Geometry: final body of the model. Coordinates: model frame, mm. Face numbers are marked on the shaded views. Round coordinates to 2 decimals unless told otherwise and drop trailing zeros. Order: outer loops, then holes, each group sorted by start corner. A loop starts at its lowest first (then second) coordinate and runs counter-clockwise, first axis right, second up. Notation, with made-up numbers: (-4, -3.75) -> (4, -3.75) arc R28 cw to (4, 17.25) -> close; hole circle Ø3 at (56.25, -30.75). An arc over 180 degrees is marked (long way). Put each result on its own line as item: value.
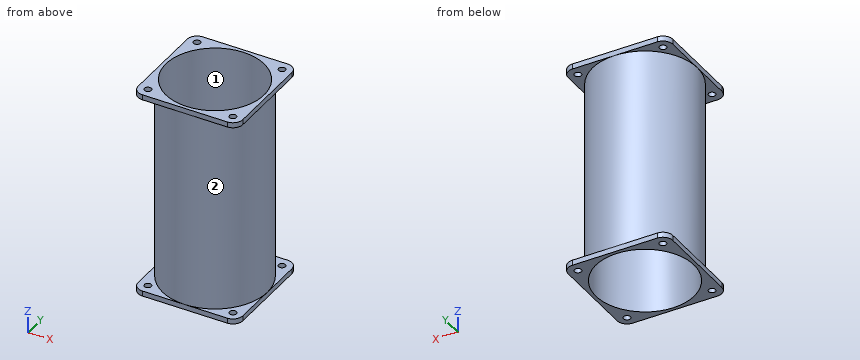
Autodesk Inventor part; units mm, degrees
ref_plane "YZ Plane" through (0, 0, 0) normal (1, 0, 0) x (0, 1, 0)
ref_plane "XZ Plane" through (0, 0, 0) normal (0, 1, 0) x (-1, 0, 0)
ref_plane "XY Plane" through (0, 0, 0) normal (0, 0, 1) x (1, 0, 0)
sketch "Skizze1" plane through (0, 0, 0) normal (0, 1, 0) x (-1, 0, 0)
  line L0 (0, 0) -> (80, 0)
  line L1 (80, 0) -> (80, -152)
  line L2 (80, -152) -> (0, -152)
  line L3 (0, -152) -> (0, 0)
  line L4 (80, -152) -> (-80, -152)
  line L5 (-80, -152) -> (-80, -160)
  line L6 (-80, -160) -> (80, -160)
  line L7 (80, -160) -> (80, -152)
  dimension "d0" = 160
  dimension "d1" = 160
  dimension "d2" = 8
revolve "Umdrehung1" add sketch "Skizze1" angle 360 about axis through (0, 0, -152) along (0, 0, 1) contours L0 L1 L2 L3
extrude "Extrusion1" add sketch "Skizze1" along normal mid plane 160 contours L2 L7 L6 L5 L4
fillet "Rundung1" radius 15 4 edges at (80, 80, -156) (-80, 80, -156) (80, -80, -156) (-80, -80, -156)
sketch "Skizze2" plane through (65, 80, -160) normal (0, 0, -1) x (-1, 0, 0)
  circle A0 centre (65, -80) radius 80
hole "Bohrung1" at (0, 0, -160) direction (0, 0, 1) diameter 150 end through all
sketch "Skizze3" plane through (65, 80, -160) normal (0, 0, -1) x (-1, 0, 0)
  line L0 (130, -145) -> (0, -145)
  line L1 (0, -145) -> (0, -15)
  line L2 (0, -15) -> (130, -15)
  line L3 (130, -15) -> (130, -145)
  line L4 (130, -145) -> (0, -15) construction
  line L5 (0, -145) -> (130, -15) construction
  point P0 (65, -80)
  dimension "d14" = 130
  dimension "d15" = 130
hole "Bohrung2" at (-65, 65, -160) at (65, 65, -160) at (65, -65, -160) at (-65, -65, -160) direction (0, 0, 1) diameter 10.5 end through all
mirror "Spiegeln1" about plane through (-80, 0, 0) normal (0, 0, 1)
equation "\"d4\" = d0"
properties part number "Gehäuse" material "Stahl AISI 1080"
1. Cut plane B-B on y = -31.5. Return loops of the section in (x, z), and give its area (3 significant figures).
Ans:
outline: (-80, -160) -> (-68.06, -160) -> (-68.06, 160) -> (-80, 160) -> (-80, 152) -> (-73.54, 152) -> (-73.54, -152) -> (-80, -152) -> close; (68.06, -160) -> (80, -160) -> (80, -152) -> (73.54, -152) -> (73.54, 152) -> (80, 152) -> (80, 160) -> (68.06, 160) -> close
area: 3,710 mm²
2. Contact query for flat-ended pins moving along their axis: P1, Ø1.5, axis at x = 12, z = -79, coming from the -Y side; P2, Ø8, axis at x = 46, z = -113.5, coming from the +Y side; P3, Ø6.5, axis at x = -65, y = -65, coming from the -Z side; P4, Ø2, axis at x = 38, z = -70.5, coming from the +Y side. Output: stop coordinate, or through.
Ans:
P1: y = -79.21
P2: y = 68.09
P3: through
P4: y = 70.93
3. Cut plane C-C on z = 116.5. Return loops of the section in (x, y), and give its area (3 significant figures).
Ans:
outline: circle Ø160 at (0, 0); hole circle Ø150 at (0, 0)
area: 2,430 mm²
4. Material intervals for probe 1 along Y at (x, z) = (65, 154.5); probe 2 along Z at (x, y) = (-58.5, -68), sorted ascending.
Ans:
probe 1: -80 to -70.25, -59.75 to -37.42, 37.42 to 59.75, 70.25 to 80
probe 2: -160 to -152, 152 to 160
5. Draft query along X for the marked faces 1 and 2. Return one class per face: +X half, -X half, draft (parallel to the pull), parting line (faces both ways), or undercut.
Ans:
face 1: undercut
face 2: parting line
6. Cut plane A-A on x = -9.5. Return loops of the section in (y, z), and give its area (3 significant figures).
Ans:
outline: (-80, -160) -> (-74.4, -160) -> (-74.4, 160) -> (-80, 160) -> (-80, 152) -> (-79.43, 152) -> (-79.43, -152) -> (-80, -152) -> close; (74.4, -160) -> (80, -160) -> (80, -152) -> (79.43, -152) -> (79.43, 152) -> (80, 152) -> (80, 160) -> (74.4, 160) -> close
area: 3,240 mm²
